from build123d import *

# Parameters (mm, degrees)
SKETCH1_W            = 94
SKETCH1_H            = 48
BOSS_EXTRUDE1_DEPTH  = 4
SKETCH8_W            = 94
SKETCH8_H            = 48
BOSS_EXTRUDE2_DEPTH  = 21
CUT_EXTRUDE1_DEPTH   = 16
SKETCH10_W           = 94
SKETCH10_H           = 48
BOSS_EXTRUDE3_DEPTH  = 5
SKETCH15_W           = 70
SKETCH15_H           = 1.5
SKETCH15_H_2         = 3
BOSS_EXTRUDE6_DEPTH  = 4
SKETCH16_W           = 94
SKETCH16_H           = 48
SKETCH16_W_2         = 84
SKETCH16_H_2         = 43
BOSS_EXTRUDE7_DEPTH  = 18
CUT_EXTRUDE4_DEPTH   = 8
SKETCH18_W           = 2
SKETCH18_H           = 20
BOSS_EXTRUDE8_DEPTH  = 6
BOSS_EXTRUDE9_DEPTH  = 4
BOSS_EXTRUDE10_DEPTH = 4
SKETCH22_W           = 14
SKETCH22_H           = 16
CUT_EXTRUDE6_DEPTH   = 3
CUT_EXTRUDE8_DEPTH   = 13.2


with BuildPart() as part:
    # Sketch1 → Boss-Extrude1 (new body)
    with BuildSketch(Plane(origin=(0, 0, 0), x_dir=(1, 0, 0), z_dir=(0, 1, 0))):
        Rectangle(SKETCH1_W, SKETCH1_H)
    extrude(amount=BOSS_EXTRUDE1_DEPTH)

    # Sketch8 → Boss-Extrude2 (add)
    with BuildSketch(Plane(origin=(0, 0, 0), x_dir=(-1, 0, 0), z_dir=(0, -1, 0))):
        Rectangle(SKETCH8_W, SKETCH8_H)
        Polygon((34, -16), (-31, -16), (-31, 6), (-39, 6), (-39, 19), (-31, 19), (-31, 16), (34, 16), align=None, mode=Mode.SUBTRACT)
    extrude(amount=BOSS_EXTRUDE2_DEPTH)

    # Sketch9 → Cut-Extrude1 (cut)
    with BuildSketch(Plane(origin=(47, 0, 0), x_dir=(0, 0, -1), z_dir=(1, 0, 0))):
        with BuildLine():
            Line((-8.547025015, -3.603370842), (-8.547025015, -15.588001804))
            ThreePointArc((-8.547025015, -15.588001804), (-12.273512507, -19.314489297), (-16, -15.588001804))
            Line((-16, -15.588001804), (-16, -3.603370842))
            ThreePointArc((-16, -3.603370842), (-12.273512507, 0.12311665), (-8.547025015, -3.603370842))
        make_face()
    extrude(amount=-CUT_EXTRUDE1_DEPTH, mode=Mode.SUBTRACT)

    # Sketch10 → Boss-Extrude3 (add)
    with BuildSketch(Plane.XZ.offset(21)):
        Rectangle(SKETCH10_W, SKETCH10_H)
        Polygon((31, -6), (39, -6), (39, -19), (-39, -19), (-39, 21), (31, 21), align=None, mode=Mode.SUBTRACT)
    extrude(amount=BOSS_EXTRUDE3_DEPTH)

    # Sketch15 → Boss-Extrude6 (add)
    with BuildSketch(Plane.XZ.offset(21)):
        with Locations((-4, 20.25)):
            Rectangle(SKETCH15_W, SKETCH15_H)
        with Locations((-4, -17.5)):
            Rectangle(SKETCH15_W, SKETCH15_H_2)
    extrude(amount=BOSS_EXTRUDE6_DEPTH)

    # Sketch16 → Boss-Extrude7 (add)
    with BuildSketch(Plane.XZ.offset(26)):
        Rectangle(SKETCH16_W, SKETCH16_H)
        with Locations((1, -0.5)):
            Rectangle(SKETCH16_W_2, SKETCH16_H_2, mode=Mode.SUBTRACT)
    extrude(amount=BOSS_EXTRUDE7_DEPTH)

    # Sketch17 → Cut-Extrude4 (cut)
    with BuildSketch(Plane.ZY.offset(47)):
        with BuildLine():
            Line((13.36, -37.297738986), (13.36, -25.248584525))
            ThreePointArc((13.36, -25.248584525), (15, -23.608584525), (16.64, -25.248584525))
            Line((16.64, -25.248584525), (16.64, -37.297738986))
            ThreePointArc((16.64, -37.297738986), (15, -38.937738986), (13.36, -37.297738986))
        make_face()
        with BuildLine():
            Line((10.64, -37.297738986), (10.64, -25.248584525))
            ThreePointArc((10.64, -25.248584525), (9, -23.608584525), (7.36, -25.248584525))
            Line((7.36, -25.248584525), (7.36, -37.297738986))
            ThreePointArc((7.36, -37.297738986), (9, -38.937738986), (10.64, -37.297738986))
        make_face()
        with BuildLine():
            Line((4.64, -37.297738986), (4.64, -25.248584525))
            ThreePointArc((4.64, -25.248584525), (3, -23.608584525), (1.36, -25.248584525))
            Line((1.36, -25.248584525), (1.36, -37.297738986))
            ThreePointArc((1.36, -37.297738986), (3, -38.937738986), (4.64, -37.297738986))
        make_face()
        with BuildLine():
            Line((-1.36, -37.297738986), (-1.36, -25.248584525))
            ThreePointArc((-1.36, -25.248584525), (-3, -23.608584525), (-4.64, -25.248584525))
            Line((-4.64, -25.248584525), (-4.64, -37.297738986))
            ThreePointArc((-4.64, -37.297738986), (-3, -38.937738986), (-1.36, -37.297738986))
        make_face()
        with BuildLine():
            Line((-7.36, -37.297738986), (-7.36, -25.248584525))
            ThreePointArc((-7.36, -25.248584525), (-9, -23.608584525), (-10.64, -25.248584525))
            Line((-10.64, -25.248584525), (-10.64, -37.297738986))
            ThreePointArc((-10.64, -37.297738986), (-9, -38.937738986), (-7.36, -37.297738986))
        make_face()
        with BuildLine():
            Line((-13.36, -37.297738986), (-13.36, -25.248584525))
            ThreePointArc((-13.36, -25.248584525), (-15, -23.608584525), (-16.64, -25.248584525))
            Line((-16.64, -25.248584525), (-16.64, -37.297738986))
            ThreePointArc((-16.64, -37.297738986), (-15, -38.937738986), (-13.36, -37.297738986))
        make_face()
    extrude(amount=-CUT_EXTRUDE4_DEPTH, mode=Mode.SUBTRACT)

    # Sketch18 → Boss-Extrude8 (add)
    with BuildSketch(Plane.XZ.offset(44)):
        with Locations((-46, 0)):
            Rectangle(SKETCH18_W, SKETCH18_H)
    extrude(amount=BOSS_EXTRUDE8_DEPTH)

    # Sketch19 → Boss-Extrude9 (add)
    with BuildSketch(Plane(origin=(-45, 0, 0), x_dir=(0, 0, -1), z_dir=(1, 0, 0))):
        Polygon((-5.55, -44), (5.55, -44), (7.8, -48), (-7.8, -48), align=None)
    extrude(amount=BOSS_EXTRUDE9_DEPTH)

    # Sketch20 → Boss-Extrude10 (add)
    with BuildSketch(Plane(origin=(47, 0, 0), x_dir=(0, 0, -1), z_dir=(1, 0, 0))):
        Polygon((3.6, -44), (9.3, -44), (11.75, -48), (1.15, -48), align=None)
        Polygon((-3.6, -44), (-1.15, -48), (-11.75, -48), (-9.3, -44), align=None)
    extrude(amount=-BOSS_EXTRUDE10_DEPTH)

    # Sketch22 → Cut-Extrude6 (cut)
    with BuildSketch(Plane.XY.offset(24)):
        with Locations((22, -36)):
            Rectangle(SKETCH22_W, SKETCH22_H)
    extrude(amount=-CUT_EXTRUDE6_DEPTH, mode=Mode.SUBTRACT)

    # Sketch28 → Cut-Extrude8 (cut)
    with BuildSketch(Plane(origin=(0, -44, 0), x_dir=(-1, 0, 0), z_dir=(0, -1, 0))):
        Polygon((-8.5, -24), (-8.5, -22.5), (-9.5, -22.5), (-9.5, -21), (12.5, -21), (12.5, -22.5), (11.5, -22.5), (11.5, -24), align=None)
    extrude(amount=-CUT_EXTRUDE8_DEPTH, mode=Mode.SUBTRACT)


solid = part.part
Read the model definition and answer for the solid it produces. Units are mm, in the model's axes. A direction names the side the tool comes from. Round coordinates to 2 decimals unless told otherwise and drop trailing zeros. Loops run counter-clockwise (first coordinate to the right, second up) from the corner with the lowest first, then second, coordinate; pieces in that order, holes last. Notation, with made-up numbers: (51.25, -30.75) - (100.25, -30.75) arc R17 cw to (100.25, -16.75) - close; hole circle Ø10 at (-29, 82.5). An arc over 180 degrees is marked (long way). One line per question, with ' | ' between items. Start each with the question number.
Q1. Section C-C on z = 0 is taken. Give the vertices of the cut face in (x, y), plus the area to 3 significant figures.
Q2. Section A-A on z = -15 is taken. Give the vertices of the cut face in (x, y), plus the area to 3 significant figures.
Q3. For faces 1 (the flat face through (-44, -31, -16.64)), 2 (the flat face through (31, -0.9, 15.3)), 3 (the flat face through (7, -11, 16)), determine the directions among +Z, -Z, +X, -X, +Y, -Y from which every point of the face is accessible in a straight line to the end or side of a thin tool.
Q4. Flat-ended cylindrical pins translate along their axes: pin 1 (4 mm diameter, centred on x = 10, z = -11.5, fed in from -Y); pin 2 (2 mm diameter, centred on x = -39.5, z = 6.5, fed in from -Y); pin 3 (1.6 mm diameter, centred on x = -40.5, z = 0, fed in from -Y). Find the tip coordinate at first contact, or state that the pin passes through.
Q5. Section B-B on x = 30 is taken. Give the vertices of the cut face in (y, z), plus the area to 3 significant figures.
Q6. Find the intervals of material crossed by L1, parallel to Z at x = 3, y = -17; L2, parallel to X at y = -17, z = -15; L3, parallel to X at y = -10.5, z = 6, in increasing order.
Q7. For a pull along X with two mould halves and no side action, classify faces 4 (the flat face through (42, -44, 22)), 5 (the flat face through (2, 0, -2)) as +X half, -X half, draft (parallel to the pull), parting line (faces both ways), or undercut.
Q8. Section D-D on y = -10 is taken. Give the vertices of the cut face in (x, z), plus the area to 3 significant figures.
Established:
1) outline: (-47, -50) - (-45, -50) - (-45, -48) - (-41, -48) - (-41, -26) - (-39, -26) - (-39, -21) - (-34, -21) - (-34, 0) - (31, 0) - (31, -26) - (43, -26) - (43, -44) - (47, -44) - (47, 4) - (-47, 4) - close | area: 1,310 mm²
2) outline: (-47, -44) - (-41, -44) - (-41, -38.94) - (-47, -38.94) - close; (-47, -23.61) - (-39, -23.61) - (-39, -21) - (-34, -21) - (-34, 0) - (39, 0) - (39, -26) - (43, -26) - (43, -44) - (47, -44) - (47, 4) - (-47, 4) - close | area: 980 mm²
3) face 1: -X | face 2: -Y | face 3: none
4) pin 1: y = 0 | pin 2: y = -26 | pin 3: y = -48
5) outline: (-44, -24) - (4, -24) - (4, 24) - (-44, 24) - (-44, 21) - (-25, 21) - (-25, 19.5) - (-21, 19.5) - (-21, 16) - (0, 16) - (0, -16) - (-25, -16) - (-25, -19) - (-26, -19) - (-26, -22) - (-44, -22) - close | area: 676 mm²
6) L1: -24 to -16, 16 to 24 | L2: -47 to -34, 39 to 47 | L3: -47 to -34, 31 to 47
7) face 4: draft | face 5: undercut
8) outline: (-47, -24) - (47, -24) - (47, 8.55) - (31, 8.55) - (31, -6) - (39, -6) - (39, -19) - (31, -19) - (31, -16) - (-34, -16) - (-34, 16) - (47, 16) - (47, 24) - (-47, 24) - close | area: 2,210 mm²
